Verification items for the finished model (mm, model axes). A direction names the side the tool comes from. Give positions to 0.01 mm unless a question says otherwise; leave off trailing zeros. Loops run counter-clockwise (first coordinate to the right, second up) from the corner with the lowest first, then second, coordinate; pieces in that order, holes last. Notation, with made-up numbers: (-13, 15) - (-2, 15) arc R10 cw to (-2, 28) - close; hole circle Ø4 at (56, -39). An arc over 180 degrees is marked (long way). One line per item, written item: value. Start each with the question number.
1. Gauge pin test, flat ends, axial feed: pin 1 (20.5 mm diameter, centred on x = 0, z = 0, fed in from -Y); pin 2 (4 mm diameter, centred on y = -0.5, z = 15, fed in from +X); pin 3 (1.5 mm diameter, centred on y = 3, z = -7, fed in from -X); pin 4 (6 mm diameter, centred on x = 2.5, z = 5, fed in from +Y). Record the tip position at first contact, or that the pin passes through.
2. Sectioned sample at D-D (z = -16.5). Record the cut outline in (x, y).
3. Mould release check, pull along X, two halves, no side actions. Record for faces 3 (the flat face through (9, 7, -10)), 4 (the cylindrical face through (-13.219, 5.232, 6.875)), 5 (the cylindrical face through (-1.612, -2.76, 2.103)), 6 (the flat face through (2, -2, -1)): pulls with the +X half, pulls with the -X half, needs draft (parallel to the pull), parting line crosses it, or undercut.
4. Access from +Z, -Z, +X, -X, +Y, -Y to the whole of each face (thin tool, end or side, straight path). Record for faces 1 (the cylindrical face through (-12.593, 5.479, -2.796)), 2 (the flat face through (-4, -4, 0)).
5. Sectioned sample at C-C (y = 1.5). Record the cut outline in (x, z).
6. Scan lines: L1, parallel to X at y = 2.65, z = 0; L2, parallel to X at y = 6.35, z = 0; L3, parallel to Y at x = 6, z = 14. Record each from-to range of solid material in increasing order. Write a range as [from, to].
from build123d import *

# Parameters (mm, degrees)
SKETCH1_R           = 21
SKETCH1_R_2         = 2
BOSS_EXTRUDE1_DEPTH = 4
SKETCH2_R           = 14.9
SKETCH2_R_2         = 12.9
BOSS_EXTRUDE2_DEPTH = 3
CHAMFER1_SIZE       = 0.5
BOSS_EXTRUDE3_START = 4
SKETCH3_R           = 21
SKETCH3_R_2         = 2.65
BOSS_EXTRUDE3_DEPTH = 4
BOSS_EXTRUDE4_START = 2
SKETCH4_R           = 2.65
SKETCH4_R_2         = 2
BOSS_EXTRUDE4_DEPTH = 2
CHAMFER2_SIZE       = 0.5


with BuildPart() as part:
    # Sketch1 → Boss-Extrude1 (new body)
    with BuildSketch(Plane(origin=(0, 0, 0), x_dir=(1, 0, 0), z_dir=(0, 1, 0))):
        with Locations(Location((0, 0, 0), (0, 0, 270))):
            Circle(SKETCH1_R)
        with Locations(Location((0, 0, 0), (0, 0, 270))):
            Circle(SKETCH1_R_2, mode=Mode.SUBTRACT)
    extrude(amount=BOSS_EXTRUDE1_DEPTH)

    # Sketch2 → Boss-Extrude2 (add)
    with BuildSketch(Plane(origin=(0, 4, 0), x_dir=(1, 0, 0), z_dir=(0, 1, 0))):
        with Locations(Location((0, 0, 0), (0, 0, 270))):
            Circle(SKETCH2_R)
        with Locations(Location((0, 0, 0), (0, 0, 270))):
            Circle(SKETCH2_R_2, mode=Mode.SUBTRACT)
    extrude(amount=BOSS_EXTRUDE2_DEPTH)

    # Chamfer1
    chamfer1_edges = [part.edges().sort_by_distance(p)[0] for p in [
        (0, 7, -14.9),
    ]]
    chamfer(chamfer1_edges, length=CHAMFER1_SIZE)

    # Sketch3 → Boss-Extrude3 (add)
    with BuildSketch(Plane.XZ.offset(BOSS_EXTRUDE3_START)):
        with Locations(Location((0, 0, 0), (0, 0, 270))):
            Circle(SKETCH3_R)
        with Locations(Location((0, 0, 0), (0, 0, 270))):
            Circle(SKETCH3_R_2, mode=Mode.SUBTRACT)
    extrude(amount=-BOSS_EXTRUDE3_DEPTH)

    # Sketch4 → Boss-Extrude4 (add)
    with BuildSketch(Plane.XZ.offset(BOSS_EXTRUDE4_START)):
        with Locations(Location((0, 0, 0), (0, 0, 270))):
            Circle(SKETCH4_R)
        with Locations(Location((0, 0, 0), (0, 0, 270))):
            Circle(SKETCH4_R_2, mode=Mode.SUBTRACT)
    extrude(amount=-BOSS_EXTRUDE4_DEPTH)

    # Chamfer2
    chamfer2_edges = [part.edges().sort_by_distance(p)[0] for p in [
        (0, -4, 2.65),
    ]]
    chamfer(chamfer2_edges, length=CHAMFER2_SIZE)


solid = part.part
Results are:
1. pin 1: stops at y = -4
1. pin 2: stops at x = 16.49
1. pin 3: stops at x = -20.05
1. pin 4: stops at y = 4
2. outline: (-12.99, -4) - (12.99, -4) - (12.99, 4) - (-12.99, 4) - close
3. face 3: needs draft
3. face 4: parting line crosses it
3. face 5: undercut
3. face 6: undercut
4. face 1: +Y
4. face 2: +Z, -Z, +X, -X, -Y
5. outline: circle Ø42 at (0, 0); hole circle Ø4 at (0, 0)
6. L1: x = [-21, -2], [2, 21]
6. L2: x = [-14.9, -12.9], [12.9, 14.9]
6. L3: y = [-4, 4]
